```python
from build123d import *

# Parameters (mm, degrees)
SKETCH1_W            = 80
SKETCH1_H            = 80
BOSS_EXTRUDE1_DEPTH  = 25.5
SKETCH2_R            = 35.75
CUT_EXTRUDE2_DEPTH   = 28
BOSS_EXTRUDE2_START  = -2
BOSS_EXTRUDE2_DEPTH  = 2
CIRPATTERN2_COUNT    = 4
SKETCH5_R            = 15
BOSS_EXTRUDE3_DEPTH  = 2
SKETCH6_R            = 3
BOSS_EXTRUDE4_DEPTH  = 17.5
FILLET1_R            = 1.5
SKETCH7_R            = 70
SKETCH7_R_2          = 38
CUT_EXTRUDE4_DEPTH   = 18
FILLET2_R            = 5
BOSS_EXTRUDE5_START  = -20
BOSS_EXTRUDE5_DEPTH  = 20
CIRPATTERN3_COUNT    = 4
SKETCH9_R            = 2.25
CUT_EXTRUDE5_DEPTH   = 37
LPATTERN1_COUNT      = 2
LPATTERN1_PITCH      = 71.5
LPATTERN1_COUNT_DIR2 = 2
LPATTERN1_PITCH_DIR2 = 71.5
CHAMFER2_SIZE        = 3
CUT_EXTRUDE6_DEPTH   = 1
CUT_EXTRUDE7_DEPTH   = 7
SCALE1_SCALE         = 1.5


with BuildPart() as part:
    # Sketch1 → Boss-Extrude1 (new body)
    with BuildSketch(Plane(origin=(0, 0, 0), x_dir=(1, 0, 0), z_dir=(0, 1, 0))):
        Rectangle(SKETCH1_W, SKETCH1_H)
    extrude(amount=BOSS_EXTRUDE1_DEPTH)

    # Sketch2 → Cut-Extrude2 (cut)
    with BuildSketch(Plane(origin=(0, 25.5, 0), x_dir=(1, 0, 0), z_dir=(0, 1, 0))):
        with Locations(Location((0, 0, 0), (0, 0, 270))):
            Circle(SKETCH2_R)
    extrude(amount=-CUT_EXTRUDE2_DEPTH, mode=Mode.SUBTRACT)

    # Sketch4 → Boss-Extrude2 (add)
    with BuildSketch(Plane.XZ.offset(BOSS_EXTRUDE2_START)):
        with BuildLine():
            Line((-1.75, 0), (0, 1.785533906))
            Line((0, 1.785533906), (-24.370530875, 26.156064781))
            ThreePointArc((-24.370530875, 26.156064781), (-25.270176953, 25.287954776), (-26.138919431, 24.388919431))
            Line((-26.138919431, 24.388919431), (-1.75, 0))
        make_face()
    boss_extrude2 = extrude(amount=BOSS_EXTRUDE2_DEPTH)

    # CirPattern2: Boss-Extrude2 ×4 about axis
    cirpattern2_axis = Axis((0, 0, 0), (0, 1, 0))
    for i in range(1, CIRPATTERN2_COUNT):
        add(boss_extrude2.rotate(cirpattern2_axis, i * 360 / CIRPATTERN2_COUNT))

    # Sketch5 → Boss-Extrude3 (add)
    with BuildSketch(Plane.XZ):
        Circle(SKETCH5_R)
    extrude(amount=-BOSS_EXTRUDE3_DEPTH)

    # Sketch6 → Boss-Extrude4 (add)
    with BuildSketch(Plane(origin=(0, 2, 0), x_dir=(1, 0, 0), z_dir=(0, 1, 0))):
        with Locations(Location((0, 0, 0), (0, 0, 90))):
            Circle(SKETCH6_R)
    extrude(amount=BOSS_EXTRUDE4_DEPTH)

    # Fillet1
    fillet1_edges = [part.edges().sort_by_distance(p)[0] for p in [
        (0, 19.5, 3),
    ]]
    fillet(fillet1_edges, radius=FILLET1_R)

    # Sketch7 → Cut-Extrude4 (cut)
    with BuildSketch(Plane.XZ.offset(-4)):
        Circle(SKETCH7_R)
        with Locations(Location((0, 0, 0), (0, 0, 270))):
            Circle(SKETCH7_R_2, mode=Mode.SUBTRACT)
    extrude(amount=-CUT_EXTRUDE4_DEPTH, mode=Mode.SUBTRACT)

    # Fillet2
    fillet2_edges = [part.edges().sort_by_distance(p)[0] for p in [
        (-40, 2, -40),
        (40, 2, -40),
        (40, 2, 40),
        (-40, 2, 40),
        (-40, 23.75, -40),
        (40, 23.75, -40),
        (40, 23.75, 40),
        (-40, 23.75, 40),
    ]]
    fillet(fillet2_edges, radius=FILLET2_R)

    # Sketch8 → Boss-Extrude5 (add)
    with BuildSketch(Plane.XZ.offset(-4).offset(BOSS_EXTRUDE5_START)):
        with BuildLine():
            Line((-3, 40), (3, 40))
            Line((3, 40), (3, 35.623903492))
            ThreePointArc((3, 35.623903492), (0, 35.75), (-3, 35.623903492))
            Line((-3, 35.623903492), (-3, 40))
        make_face()
    boss_extrude5 = extrude(amount=BOSS_EXTRUDE5_DEPTH)

    # CirPattern3: Boss-Extrude5 ×4 about axis
    cirpattern3_axis = Axis((0, 0, 0), (0, 1, 0))
    for i in range(1, CIRPATTERN3_COUNT):
        add(boss_extrude5.rotate(cirpattern3_axis, i * 360 / CIRPATTERN3_COUNT))

    # Sketch9 → Cut-Extrude5 (cut)
    with BuildSketch(Plane(origin=(0, 25.5, 0), x_dir=(-1, 0, 0), z_dir=(0, 1, 0))):
        with Locations(Location((35.75, -35.75, 0), (0, 0, 90))):
            Circle(SKETCH9_R)
    cut_extrude5 = extrude(amount=-CUT_EXTRUDE5_DEPTH, mode=Mode.SUBTRACT)

    # LPattern1: Cut-Extrude5 2 × 2
    with Locations(*[(i * LPATTERN1_PITCH, 0, j * LPATTERN1_PITCH_DIR2) for i in range(LPATTERN1_COUNT) for j in range(LPATTERN1_COUNT_DIR2) if (i, j) != (0, 0)]):
        add(cut_extrude5, mode=Mode.SUBTRACT)

    # Chamfer2
    chamfer2_edges = [part.edges().sort_by_distance(p)[0] for p in [
        (0, 25.5, -35.75),
    ]]
    chamfer(chamfer2_edges, length=CHAMFER2_SIZE)

    # Sketch11 → Cut-Extrude6 (cut)
    with BuildSketch(Plane.XZ):
        Polygon((-28.863216429, 27.820323211), (-7.554875149, 6.51198193), (-6.494214977, 7.572642102), (-28.241896086, 29.320323211), (-40, 29.320323211), (-40, 27.820323211), align=None)
    extrude(amount=-CUT_EXTRUDE6_DEPTH, mode=Mode.SUBTRACT)

    # Sketch12 → Cut-Extrude7 (cut)
    with BuildSketch(Plane.XZ.offset(-1)):
        Polygon((-6.494214977, 7.572642102), (-7.554875149, 8.633302273), (-8.61553532, 7.572642102), (-7.554875149, 6.51198193), align=None)
    extrude(amount=-CUT_EXTRUDE7_DEPTH, mode=Mode.SUBTRACT)


with BuildPart() as part_1:
    # Scale1: scaled about (0.049360087, 11.297047604, -0.045989388)
    add(part.part.scale(SCALE1_SCALE).moved(Location((-0.024680043, -5.648523802, 0.022994694))))


solid = part_1.part
```
Check sheet for the modelled part. Datum: model origin and axes. Units: mm. A direction names the side the tool comes from. Round coordinates to 2 decimals unless told otherwise and drop trailing zeros. Order: outer loops, then holes, each group sorted by start corner. A loop starts at its lowest first (then second) coordinate and runs counter-clockwise, first axis right, second up.
1) Mould release check, pull along Y, two halves, no side actions. Record for faces 6 (the flat face through (-34, -4.149, 33)), 7 (the flat face through (58, 14, 4.523)), 8 (the cylindrical face through (57.72, 30.01, -57.84)), 9 (the flat face through (-23, 32.601, -54)): +Y half, -Y half, draft (parallel to the pull), parting line (faces both ways), or undercut.
2) Go/stop test with flat-tipped pins: pin 1 Ø0.8 at (x, y) = (-55.5, -5) entering from -Z; pin 2 Ø4 at (y, z) = (20, -39) entering from +X; pin 3 Ø2 at (y, z) = (15, 19) entering from -X; pin 4 Ø6 at (x, z) = (-53.65, -53.6) entering from -Y. Record where each tip stops, or that it passes through.
3) Scan lines: line 1 (X direction, y = -3, z = -24.5); line 2 (Y direction, x = -53, z = -26.5); line 3 (Z direction, x = -27, y = 23.5). Record each from-to range of solid material in increasing order.
4) Tool access check on faces 1 (the flat face through (-28.084, -4.128, -25.358)), 2 (the cylindrical face through (40.677, 13.662, 39.928)), 3 (the conical face through (-37.766, 28.383, -38.467)), 4 (the flat face through (-4.525, 14, -58)), 5 (the cylindrical face through (-39.929, 13.662, 40.725)). Record the directions out of +Z, -Z, +X, -X, +Y, -Y that give a thin tool (end or side, any length) a straight path to the whole face; none if there is none.
5) Section check A-A (y = 12.5). Record the boundary of the cut face in (x, z) (3 decimals).
6) Section check B-B (x = 10.5). Give the number of separate pieces and of enclosed holes in the cut face, and give its area (3 significant figures).
Result:
1. face 6: -Y half
1. face 7: undercut
1. face 8: draft
1. face 9: +Y half
2. pin 1: stops at z = -59.52
2. pin 2: stops at x = 43.31
2. pin 3: stops at x = -54.12
2. pin 4: passes through
3. line 1: x = -60.02 to -47.71, -27.23 to -21.92, 21.82 to 27.12, 47.66 to 59.98
3. line 2: y = -5.65 to 0.35, 27.35 to 32.6
3. line 3: z = -50.19 to -46.32, 46.37 to 50.24
4. face 1: +Y, -Y
4. face 2: +Z, +X
4. face 3: +Y
4. face 4: -Z, -X
4. face 5: +Z, -X
5. outline: (-60.025, -4.477) - (-56.847, -4.477) arc R57 ccw to (-4.525, -56.799) - (-4.525, -59.977) - (4.475, -59.977) - (4.475, -56.799) arc R57 ccw to (56.797, -4.477) - (59.975, -4.477) - (59.975, 4.523) - (56.797, 4.523) arc R57 ccw to (4.475, 56.845) - (4.475, 60.023) - (-4.525, 60.023) - (-4.525, 56.845) arc R57 ccw to (-56.847, 4.523) - (-60.025, 4.523) - close; circle Ø9 at (-0.025, 0.023); hole circle Ø107.25 at (-0.025, 0.023)
6. separate pieces: 3
6. enclosed holes: 0
6. area: 451 mm2
